Source: CAD feature listing. Evaluate the final solid. Frame: model axes, mm. Give positions to 0.01 mm unless a question says otherwise; leave off trailing zeros. Order: outer loops, then holes, each group sorted by start corner. A loop starts at its lowest first (then second) coordinate and runs counter-clockwise, first axis right, second up. Notation, with made-up numbers: M -40,54.25 L -36,54.25 A27 cw -36,87.25 Z; hole C 33.5,23.25 d9. An arc over 180 degrees is marked long. Answer in a Markdown table with one row per item. Add a question column.
(1) Pin query (flat end, axial travel): P1, Ø2, axis at x = 42.5, z = 3.5, coming from the -Y side; P2, Ø6, axis at y = -69, z = 1, coming from the +X side; P3, Ø2, axis at y = -47.5, z = 7.5, coming from the -X side. Return the tip coordinate at first contact, or that it passes through.
(2) Material intervals for line 1 along Y through (x, z) = (0, 3.35); line 2 along X through (y, z) = (51, 1) (3 decimals); line 3 along X through (y, z) = (-50, 8), sorted ascending.
(3) Section query C-C, the plane y = 73.5. Return loops of the section in (x, z).
from build123d import *

# Parameters (mm, degrees)
F0_R     = 88.9
F0_R_2   = 57.15
F1_DEPTH = 11.1125
F2_R     = 63.5
F3_DEPTH = 6.35
F5_D     = 6.35
F6_R     = 1.5875


with BuildPart() as f1:
    # F0 (on Top) → F1 (new body)
    with BuildSketch(Plane.XY):
        Circle(F0_R)
        Circle(F0_R_2, mode=Mode.SUBTRACT)
    extrude(amount=F1_DEPTH)

    # F2 (on Top) → F3 (cut)
    with BuildSketch(Plane.XY):
        Circle(F2_R)
    extrude(amount=F3_DEPTH, mode=Mode.SUBTRACT)

    # F5 (through all)
    with Locations(Plane(origin=(0, 0, 0), x_dir=(1, 0, 0), z_dir=(0, 0, -1))):
        with Locations((10.2400904958, 80.6323690997), (-64.7096347598, 49.1843630563), (-74.9497252556, -31.4480060434), (-10.2400904958, -80.6323690997), (64.7096347598, -49.1843630563), (74.9497252556, 31.4480060434)):
            Hole(F5_D / 2)

    # F6
    f6_edges = [f1.edges().sort_by_distance(p)[0] for p in [
        (-63.5, 0, 6.35),
    ]]
    fillet(f6_edges, radius=F6_R)


solid = f1.part
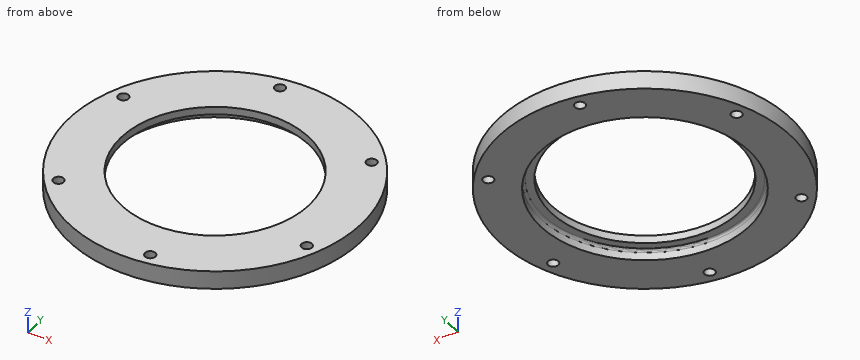
Values follow:
| question | item | result |
|---|---|---|
| 1 | P1 | stops at y = -78.62 |
| 1 | P2 | stops at x = 59.56 |
| 1 | P3 | stops at x = -75.77 |
| 2 | line 1 | y = -88.9 to -63.5, 63.5 to 88.9 |
| 2 | line 2 | x = -72.816 to -37.832, 37.832 to 62.105, 67.314 to 72.816 |
| 2 | line 3 | x = -73.51 to -67.78, -61.64 to -27.68, 27.68 to 73.51 |
| 3 | outline | M -50.01,0 L 50.01,0 L 50.01,11.11 L -50.01,11.11 Z |
